CAD build for the part. Positions are in the model's coordinates, mm. Give positions to 0.01 mm unless a question says otherwise; leave off trailing zeros. Write each loop counter-clockwise with the first axis right and the second up, starting at its lowest first coordinate (ties: lowest second). Pieces come first, ordered by that corner, then holes. Notation, with made-up numbers: (-33, -9) - (-7, -9) arc R22 cw to (-7, 11) - close; hole circle Ø8 at (67.5, 37). An arc over 180 degrees is marked (long way). Put each result on its own line as item: value. Start each with the question number.
1. Wall check: line 1 (X direction, y = 9, z = 6.25); line 2 (X direction, y = 41, z = 5); line 3 (X direction, y = 21, z = 4.5). Give the ranges that are in metal, low to high.
2. Cut at A-A on z = 5.5. List the corners of the cut face in (x, y).
3. Mould opens along Y. For faces 1 (the cylindrical face through (104.335, 9.966, 4.056)), 2 (the flat face through (10, -0.815, 4)), 3 (the flat face through (10, 49.185, 4)), 4 (the flat face through (10, 30, 8)) say: +Y half, -Y half, draft (parallel to the pull), parting line (faces both ways), or undercut.
from build123d import *

# Parameters (mm, degrees)
IZIM1_W                              = 200
IZIM1_H                              = 50
Y_KSEKLIK_EKSTR_ZYON1_DEPTH          = 8
M5_HELISARMAL_I_IN_Z_VANA_MATKAB_1_D = 5.2
M5_HELISARMAL_I_IN_Z_VANA_MATKAB_2_D = 5.2
KES_EKSTR_ZYON1_DEPTH                = 10


with BuildPart() as part:
    # Çizim1 → Yükseklik-Ekstrüzyon1 (new body)
    with BuildSketch(Plane.XY):
        with Locations((11.855409505, 24.184782609)):
            Rectangle(IZIM1_W, IZIM1_H)
    extrude(amount=Y_KSEKLIK_EKSTR_ZYON1_DEPTH)

    # M5 Helisarmal için Zıvana matkabı1 (through all)
    with Locations(Plane(origin=(0, 0, 0), x_dir=(-1, 0, 0), z_dir=(0, 0, -1))):
        with Locations((-101.855409505, 39.184782609), (-101.855409505, 9.184782609), (78.144590495, 9.184782609), (78.144590495, 39.184782609)):
            Hole(M5_HELISARMAL_I_IN_Z_VANA_MATKAB_1_D / 2)

    # M5 Helisarmal için Zıvana matkabı2 (through all)
    with Locations(Plane(origin=(71.855409505, 9.184782609, 0), x_dir=(-1, 0, 0), z_dir=(0, 0, -1))):
        with Locations((0, 0), (120, 0)):
            Hole(M5_HELISARMAL_I_IN_Z_VANA_MATKAB_2_D / 2)

    # Çizim8 → Kes-Ekstrüzyon1 (cut)
    with BuildSketch(Plane(origin=(0, 0, 0), x_dir=(-1, 0, 0), z_dir=(0, 0, -1))):
        with BuildLine():
            ThreePointArc((-7.805409505, 24.184782609), (-8.991627041, 27.048565073), (-11.855409505, 28.234782609))
            Line((-11.855409505, 28.234782609), (-11.855409505, 20.134782609))
            ThreePointArc((-11.855409505, 20.134782609), (-8.991627041, 21.321000145), (-7.805409505, 24.184782609))
        make_face()
        with BuildLine():
            Line((-11.855409505, 20.134782609), (-11.855409505, 28.234782609))
            ThreePointArc((-11.855409505, 28.234782609), (-15.905409505, 24.184782609), (-11.855409505, 20.134782609))
        make_face()
    extrude(amount=-KES_EKSTR_ZYON1_DEPTH, mode=Mode.SUBTRACT)


solid = part.part
Report:
1. line 1: x = -88.14 to -80.74, -75.55 to -50.74, -45.55 to 69.26, 74.45 to 99.26, 104.45 to 111.86
1. line 2: x = -88.14 to -80.01, -76.28 to 99.99, 103.72 to 111.86
1. line 3: x = -88.14 to 9.35, 14.36 to 111.86
2. outline: (-88.14, -0.82) - (111.86, -0.82) - (111.86, 49.18) - (-88.14, 49.18) - close; hole circle Ø5.2 at (-78.14, 9.18); hole circle Ø5.2 at (-78.14, 39.18); hole circle Ø5.2 at (-48.14, 9.18); hole circle Ø8.1 at (11.86, 24.18); hole circle Ø5.2 at (71.86, 9.18); hole circle Ø5.2 at (101.86, 9.18); hole circle Ø5.2 at (101.86, 39.18)
3. face 1: undercut
3. face 2: -Y half
3. face 3: +Y half
3. face 4: draft
